Model file for the job. Use its own axes, mm. Round coordinates to 2 decimals unless told otherwise and drop trailing zeros. Write each loop counter-clockwise with the first axis right and the second up, starting at its lowest first coordinate (ties: lowest second). Pieces come first, ordered by that corner, then holes.
```python
from build123d import *

# Parameters (mm, degrees)
SKETCH_1_W          = 262.1
SKETCH_1_H          = 166.2
EXTRUDE_1_DEPTH     = 1
SKETCH_2_R          = 1.5
SKETCH_2_W          = 8.4
SKETCH_2_H          = 16.8
SKETCH_2_W_2        = 262.1
SKETCH_2_H_2        = 0.2
SKETCH_2_W_3        = 257.1
SKETCH_2_H_3        = 1
CUT_EXTRUDE1_DEPTH  = 10
SKETCH1_R           = 1.5
CUT_EXTRUDE2_DEPTH  = 10
SKETCH2_W           = 245.3
SKETCH2_H           = 8.1
BOSS_EXTRUDE1_DEPTH = 2


with BuildPart() as part:
    # 草图1 → 凸台-拉伸1 (new, symmetric)
    with BuildSketch(Plane.XY):
        Rectangle(SKETCH_1_W, SKETCH_1_H)
    extrude(amount=EXTRUDE_1_DEPTH, both=True)

    # 草图2 → Cut-Extrude1 (cut)
    with BuildSketch(Plane.XY.offset(1)):
        with Locations((-126.85, 73.3)):
            Circle(SKETCH_2_R)
        with Locations((-126.85, 37.3)):
            Circle(SKETCH_2_R)
        with Locations((-126.85, 1.3)):
            Circle(SKETCH_2_R)
        with Locations((-126.85, -34.7)):
            Circle(SKETCH_2_R)
        with Locations((-126.85, -70.7)):
            Circle(SKETCH_2_R)
        with Locations((126.85, -70.7)):
            Circle(SKETCH_2_R)
        with Locations((126.85, -34.7)):
            Circle(SKETCH_2_R)
        with Locations((126.85, 1.3)):
            Circle(SKETCH_2_R)
        with Locations((126.85, 37.3)):
            Circle(SKETCH_2_R)
        with Locations((126.85, 73.3)):
            Circle(SKETCH_2_R)
        with Locations((-126.85, 55.1)):
            Rectangle(SKETCH_2_W, SKETCH_2_H)
        with Locations((-126.85, 19.1)):
            Rectangle(SKETCH_2_W, SKETCH_2_H)
        with Locations((-126.85, -16.9)):
            Rectangle(SKETCH_2_W, SKETCH_2_H)
        with Locations((-126.85, -52.9)):
            Rectangle(SKETCH_2_W, SKETCH_2_H)
        with Locations((126.85, -52.9)):
            Rectangle(SKETCH_2_W, SKETCH_2_H)
        with Locations((126.85, -16.9)):
            Rectangle(SKETCH_2_W, SKETCH_2_H)
        with Locations((126.85, 19.1)):
            Rectangle(SKETCH_2_W, SKETCH_2_H)
        with Locations((126.85, 55.1)):
            Rectangle(SKETCH_2_W, SKETCH_2_H)
        with Locations((0, 83.089141708)):
            Rectangle(SKETCH_2_W_2, SKETCH_2_H_2)
        with Locations((2.5, -82.6)):
            Rectangle(SKETCH_2_W_3, SKETCH_2_H_3)
    extrude(amount=-CUT_EXTRUDE1_DEPTH, mode=Mode.SUBTRACT)

    # Sketch1 → Cut-Extrude2 (cut)
    with BuildSketch(Plane.XY.offset(1)):
        with Locations((100, -70.35)):
            Circle(SKETCH1_R)
        with Locations((80, -70.35)):
            Circle(SKETCH1_R)
        with Locations((60, -70.35)):
            Circle(SKETCH1_R)
        with Locations((40, -70.35)):
            Circle(SKETCH1_R)
        with Locations((20, -70.35)):
            Circle(SKETCH1_R)
        with Locations((0, -70.35)):
            Circle(SKETCH1_R)
        with Locations((-20, -70.35)):
            Circle(SKETCH1_R)
        with Locations((-40, -70.35)):
            Circle(SKETCH1_R)
        with Locations((-60, -70.35)):
            Circle(SKETCH1_R)
        with Locations((-80, -70.35)):
            Circle(SKETCH1_R)
        with Locations((-100, -70.35)):
            Circle(SKETCH1_R)
    extrude(amount=-CUT_EXTRUDE2_DEPTH, mode=Mode.SUBTRACT)

    # Sketch2 → Boss-Extrude1 (add)
    with BuildSketch(Plane.XY.offset(1)):
        with Locations((0, 87.039141708)):
            Rectangle(SKETCH2_W, SKETCH2_H)
    extrude(amount=-BOSS_EXTRUDE1_DEPTH)


solid = part.part
```
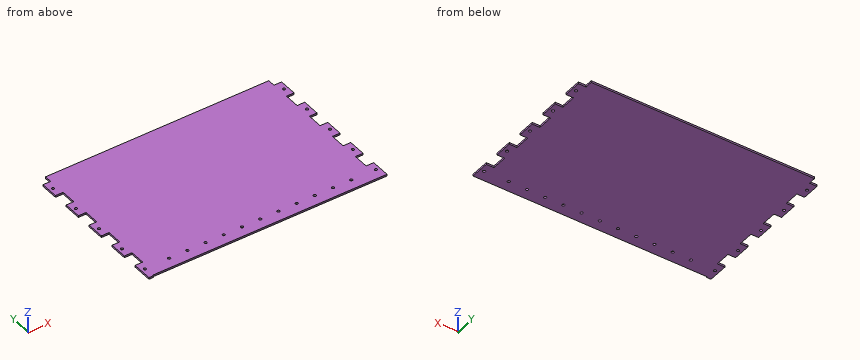
1) Flat gauge pin, fed straight in: pin 1 Ø1 at (x, z) = (129, 0.5) entering from +Y. Where does the tip first touch, or does it go through?
2) Wall check: probe 1 along Y at (x, z) = (80, -0.05); probe 2 along X at (y, z) = (72, 0.6); probe 3 along Y at (x, z) = (111.5, -0.5). Give the ranges that are in metal, low to high.
3) Cut at B-B on y = -19.5. List the corners of the cut face in (x, z).
4) Cut at A-A on z = -0.5. Give the number of separate pieces and of enclosed holes in the cut face, and give its area (3 significant figures).
Result sheet:
1. pin 1: stops at y = 82.99
2. probe 1: y = -82.1 to -71.85, -68.85 to 91.09
2. probe 2: x = -131.05 to -127.6, -126.1 to 126.1, 127.6 to 131.05
2. probe 3: y = -82.1 to 91.09
3. outline: (-122.65, -1) - (122.65, -1) - (122.65, 1) - (-122.65, 1) - close
4. separate pieces: 1
4. enclosed holes: 21
4. area: 44,000 mm2
